```python
from build123d import *

# Parameters (mm, degrees)
F0_R     = 6.4084954246
F1_DEPTH = 31.75
F3_D     = 15.875
F4_R     = 15.87499


# Not quite as in the source:
# - a fillet or chamfer is up to 0.001 mm smaller than in the source, because OpenCascade refuses the exact size


with BuildPart() as f1:
    # F0 (on Front) → F1 (new body)
    with BuildSketch(Plane.XZ):
        with BuildLine():
            Line((32.4883715089, 9.525), (-43.7116284911, 9.525))
            ThreePointArc((-43.7116284911, 9.525), (-59.5866284911, -6.35), (-43.7116284911, -22.225))
            Line((-43.7116284911, -22.225), (32.4883715089, -22.225))
            Line((32.4883715089, -22.225), (32.4883715089, -12.7))
            Line((32.4883715089, -12.7), (7.0883715089, -12.7))
            Line((7.0883715089, -12.7), (7.0883715089, 0))
            Line((7.0883715089, 0), (32.4883715089, 0))
            Line((32.4883715089, 0), (32.4883715089, 9.525))
        make_face()
        with Locations((-43.7116284911, -6.35)):
            Circle(F0_R, mode=Mode.SUBTRACT)
    extrude(amount=F1_DEPTH)

    # F3 (through all)
    with Locations(Plane.XY.offset(9.525)):
        with Locations((16.6133715089, -15.875)):
            Hole(F3_D / 2)

    # F4 (radius 15.875 in the source; OpenCascade refuses exactly that, so slightly less here)
    f4_edges = [f1.edges().sort_by_distance(p)[0] for p in [
        (32.488372, -31.75, 4.7625),
        (32.488372, 0, 4.7625),
        (32.488372, -31.75, -17.4625),
        (32.488372, 0, -17.4625),
    ]]
    fillet(f4_edges, radius=F4_R)


solid = f1.part
```
Read the model definition and answer for the solid it produces. Units are mm, in the model's axes. A direction names the side the tool comes from. Round coordinates to 2 decimals unless told otherwise and drop trailing zeros. Write each loop counter-clockwise with the first axis right and the second up, starting at its lowest first coordinate (ties: lowest second). Pieces come first, ordered by that corner, then holes. Notation, with made-up numbers: (88, -13) - (142, -13) arc R17 cw to (142, 2) - close; hole circle Ø5 at (-36, 84). An arc over 180 degrees is marked (long way). One line per item, written item: value.
Q1. Which of the six approach directions +Z, -Z, +X, -X, +Y, -Y give full straight-line access (tool end or side, diameter ignored) to faces 4 (the flat face through (26, -16, -12.7)), 5 (the cylindrical face through (27.96, -26.98, 4.83))?
The answers:
face 4: +X, +Y, -Y
face 5: +Z, -Z, +X, -Y
Q2. For a pull along Y with two mould halves and no side action, classify faces 1 (the cylindrical face through (-50.114, -15.653, -6.068)), 2 (the cylindrical face through (9.281, -18.915, -17.529)), 3 (the cylindrical face through (27.715, -4.527, -17.396)) as pulls with the +Y half, pulls with the -Y half, needs draft (parallel to the pull), parting line crosses it, or undercut.
The answers:
face 1: needs draft
face 2: undercut
face 3: pulls with the +Y half
Q3. Straight lines are drawn through the part: line 1 (Z direction, x = 25.5, y = -10) (3 decimals); line 2 (X direction, y = -8, z = -6); line 3 (X direction, y = -22, z = -5). For each, find the intervals that lie inside material, in ascending order. Write a range as from..to.
The answers:
line 1: z = -22.225..-12.7, 0..9.525
line 2: x = -59.58..-50.11, -37.31..7.09
line 3: x = -59.53..-49.98, -37.45..7.09
Q4. Find section B-B (y = -10.5). Count the separate pieces of the cut face and the enclosed holes in it, and give its area (3 significant figures).
The answers:
separate pieces: 3
enclosed holes: 1
area: 2,120 mm2
Q5. Each of these flat-tipped pins is pushed along its axis until it touches: P1, Ø10, axis at y = -27.5, z = -15.5, coming from the +X side; P2, Ø18.5, axis at x = 16.61, y = -15.88, coming from the +Z side (3 decimals); P3, Ø12, axis at y = -7.5, z = 2.5, coming from the +X side; P4, Ø9.5, axis at x = 16.61, y = -15.88, coming from the -Z side (3 decimals). Where does it stop, or does it pass through?
The answers:
P1: stops at x = 31.04
P2: stops at z = 9.525
P3: stops at x = 32.31
P4: passes through
Q6. Find section A-A (z = -6.35). Determine the outline of the cut face in (x, y).
The answers:
outline: (-59.59, -31.75) - (-50.12, -31.75) - (-50.12, 0) - (-59.59, 0) - close; (-37.3, -31.75) - (7.09, -31.75) - (7.09, 0) - (-37.3, 0) - close
